```python
from build123d import *

# Parameters (mm, degrees)
SKETCH1_R           = 29.5
BOSS_EXTRUDE1_DEPTH = 29
CUT_EXTRUDE1_DEPTH  = 51.808463862
SKETCH3_R           = 7.7
CUT_EXTRUDE2_DEPTH  = 51.808463862
SKETCH4_W           = 0.6
SKETCH4_H           = 22.211954595
SKETCH4_W_2         = 23.241543893
SKETCH4_H_2         = 0.6
CUT_EXTRUDE3_DEPTH  = 51.808464035


with BuildPart() as part:
    # Sketch1 → Boss-Extrude1 (new body)
    with BuildSketch(Plane.XY):
        with Locations(Location((0, 0, 0), (0, 0, 180))):
            Circle(SKETCH1_R)
    extrude(amount=BOSS_EXTRUDE1_DEPTH)

    # Sketch2 → Cut-Extrude1 (cut, through all)
    with BuildSketch(Plane.XY.offset(29)):
        with BuildLine():
            Line((0, 0), (29.5, 0))
            ThreePointArc((29.5, 0), (-20.859650045, 20.859650045), (0, -29.5))
            Line((0, -29.5), (0, 0))
        make_face()
    extrude(amount=-CUT_EXTRUDE1_DEPTH, mode=Mode.SUBTRACT)

    # Sketch3 → Cut-Extrude2 (cut, through all)
    with BuildSketch(Plane(origin=(0, 0, 0), x_dir=(1, 0, 0), z_dir=(0, 1, 0))):
        Circle(SKETCH3_R)
    extrude(amount=-CUT_EXTRUDE2_DEPTH, mode=Mode.SUBTRACT)

    # Sketch4 → Cut-Extrude3 (cut, through all)
    with BuildSketch(Plane(origin=(0, 0, 0), x_dir=(1, 0, 0), z_dir=(0, 1, 0))):
        with Locations((0.3, -17.894022703)):
            Rectangle(SKETCH4_W, SKETCH4_H)
        with Locations((17.879228054, -0.3)):
            Rectangle(SKETCH4_W_2, SKETCH4_H_2)
    extrude(amount=-CUT_EXTRUDE3_DEPTH, mode=Mode.SUBTRACT)


solid = part.part
```
Design review of the part built by this model. Coordinates are the model's own, in mm. Round coordinates to 2 decimals unless told otherwise and drop trailing zeros. Order: outer loops, then holes, each group sorted by start corner. A loop starts at its lowest first (then second) coordinate and runs counter-clockwise, first axis right, second up. Notation, with made-up numbers: (-24, 37.25) - (27, 37.25) arc R27 ccw to (27, 61.25) - close; hole circle Ø11 at (8.5, -25.5). An arc over 180 degrees is marked (long way). Return JSON: item names as keys, results as strings.
Q1. Consider section A-A on y = -10. Write out the cut boundary in (x, z), plus the area to 3 significant figures.
Computed values:
{"outline": "(0.6, 7.68) arc R7.7 cw to (7.68, 0.6) - (27.75, 0.6) - (27.75, 29) - (0.6, 29) - close", "area": "733 mm2"}
Q2. Consider section D-D on y = -24.75. Write out the cut boundary in (x, z), plus the area to 3 significant figures.
Computed values:
{"outline": "(0.6, 7.68) arc R7.7 cw to (7.68, 0.6) - (16.05, 0.6) - (16.05, 29) - (0.6, 29) - close", "area": "401 mm2"}
Q3. Consider section B-B on z = 27. Write out the cut boundary in (x, y), plus the area to 3 significant figures.
Computed values:
{"outline": "(0.6, -29.49) arc R29.5 ccw to (29.5, 0) - (0.6, 0) - close", "area": "666 mm2"}
Q4. For pin 1 Ø4 at (y, z) = (-7.5, 8) entering from +X; pin 2 Ø1.5 at (x, z) = (19, 23) entering from -Y; pin 3 Ø4 at (x, z) = (14.5, 20.5) entering from -Y, all flat-tipped, find the tip position at first contact; note any pin that passes through.
Computed values:
{"pin 1": "stops at x = 28.98", "pin 2": "stops at y = -23.18", "pin 3": "stops at y = -26.72"}
Q5. Wall thickness on L1, parallel to X at y = -8.75, z = 3.75; L2, parallel to X at y = -1.5, z = 15; L3, parallel to Y at x = 21.5, z = 2: over which ranges is each line inside the solid? List them lowest first. Write a range as [from, to].
Computed values:
{"L1": "x = [6.73, 28.17]", "L2": "x = [0.6, 29.46]", "L3": "y = [-20.2, 0]"}
Q6. Consider section C-C on x = 12.5. Write out the cut boundary in (y, z), plus the area to 3 significant figures.
Computed values:
{"outline": "(-26.72, 0.6) - (0, 0.6) - (0, 29) - (-26.72, 29) - close", "area": "759 mm2"}
